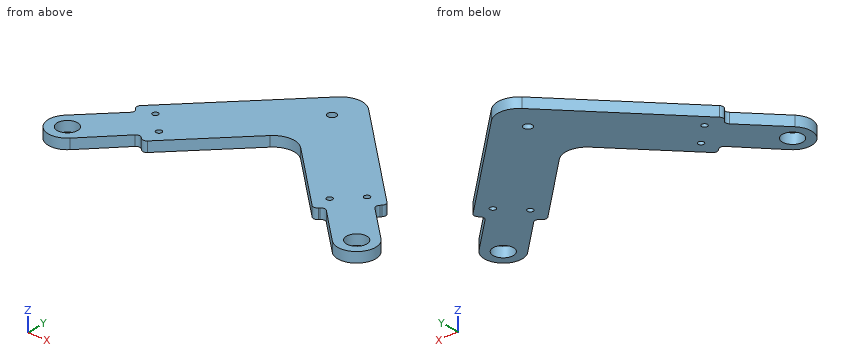
```python
from build123d import *

# Parameters (mm, degrees)
SKETCH7_R           = 3.5
SKETCH7_R_2         = 1
SKETCH7_R_3         = 1.5
BOSS_EXTRUDE1_DEPTH = 3.5
FILLET1_R           = 7.5
FILLET2_R           = 7.5
FILLET3_R           = 1.5
FILLET4_R           = 1.5
FILLET5_R           = 1.5


with BuildPart() as part:
    # Sketch7 → Boss-Extrude1 (new body)
    with BuildSketch(Plane.XY):
        with BuildLine():
            Line((-91.161165235, 18.03122292), (-104.596194078, 4.596194078))
            ThreePointArc((-104.596194078, 4.596194078), (-104.565177968, -4.627002282), (-95.342398812, -4.533955357))
            Line((-95.342398812, -4.533955357), (-82.149090724, 9.019148409))
            Line((-82.149090724, 9.019148409), (-79.493903346, 6.363961031))
            Line((-79.493903346, 6.363961031), (-50, 35.857864376))
            Line((-50, 35.857864376), (-20.445483687, 6.303348063))
            Line((-20.445483687, 6.303348063), (-17.970609953, 8.778221797))
            Line((-17.970609953, 8.778221797), (-4.596194078, -4.596194078))
            ThreePointArc((-4.596194078, -4.596194078), (4.596194078, -4.596194078), (4.596194078, 4.596194078))
            Line((4.596194078, 4.596194078), (-8.778221797, 17.970609953))
            Line((-8.778221797, 17.970609953), (-6.303348063, 20.445483687))
            Line((-6.303348063, 20.445483687), (-50, 64.142135624))
            Line((-50, 64.142135624), (-93.636038969, 20.506096654))
            Line((-93.636038969, 20.506096654), (-91.161165235, 18.03122292))
        make_face()
        Circle(SKETCH7_R, mode=Mode.SUBTRACT)
        with Locations((-100, 0)):
            Circle(SKETCH7_R, mode=Mode.SUBTRACT)
        with Locations((-86.564971157, 20.506096654)):
            Circle(SKETCH7_R_2, mode=Mode.SUBTRACT)
        with Locations((-50, 50)):
            Circle(SKETCH7_R_3, mode=Mode.SUBTRACT)
        with Locations((-13.374415875, 20.445483687)):
            Circle(SKETCH7_R_2, mode=Mode.SUBTRACT)
        with Locations((-20.445483687, 13.374415875)):
            Circle(SKETCH7_R_2, mode=Mode.SUBTRACT)
        with Locations((-79.493903346, 13.435028843)):
            Circle(SKETCH7_R_2, mode=Mode.SUBTRACT)
    extrude(amount=BOSS_EXTRUDE1_DEPTH)

    # Fillet1
    fillet1_edges = [part.edges().sort_by_distance(p)[0] for p in [
        (-50, 64.142135624, 1.75),
    ]]
    fillet(fillet1_edges, radius=FILLET1_R)

    # Fillet2
    fillet2_edges = [part.edges().sort_by_distance(p)[0] for p in [
        (-50, 35.857864376, 1.75),
    ]]
    fillet(fillet2_edges, radius=FILLET2_R)

    # Fillet3
    fillet3_edges = [part.edges().sort_by_distance(p)[0] for p in [
        (-82.149090724, 9.019148409, 1.75),
        (-93.636038969, 20.506096654, 1.75),
        (-17.970609953, 8.778221797, 1.75),
        (-20.445483687, 6.303348063, 1.75),
        (-79.493903346, 6.363961031, 1.75),
    ]]
    fillet(fillet3_edges, radius=FILLET3_R)

    # Fillet4
    fillet4_edges = [part.edges().sort_by_distance(p)[0] for p in [
        (-6.303348063, 20.445483687, 1.75),
        (-8.778221797, 17.970609953, 1.75),
    ]]
    fillet(fillet4_edges, radius=FILLET4_R)

    # Fillet5
    fillet5_edges = [part.edges().sort_by_distance(p)[0] for p in [
        (-91.161165235, 18.03122292, 1.75),
    ]]
    fillet(fillet5_edges, radius=FILLET5_R)


solid = part.part
```
Part model, mm, in its own coordinate system. Round coordinates to 2 decimals unless told otherwise and drop trailing zeros. Loops run counter-clockwise (first coordinate to the right, second up) from the corner with the lowest first, then second, coordinate; pieces in that order, holes last.
Item 1: Cut at D-D, the plane y = 37. Give the cut face in (x, z).
Item 2: Cut at C-C, the plane y = 50. Give the cut face in (x, z), then the cut area to 3 significant figures.
Item 3: Cut at B-B, the plane z = 1.9. State how many separate pieces and enclosed holes the cut face has, then the cut area to 3 significant figures.
Item 4: Drill centre lines: line 1 (X direction, y = 0.5, z = 1.45); line 2 (Y direction, x = -50, z = 1.9); line 3 (X direction, y = -2.5, z = 0.6). Where is each one in solid material? Low to high.
Item 5: Drop flat-ended pins along their axis: P1, Ø2, axis at x = -37, z = 0.5, coming from the +Y side; P2, Ø2, axis at y = 33.5, z = 3, coming from the +X side; P3, Ø2, axis at x = -86, z = 2, coming from the -Y side. Give the stop position or say it passes through.
Item 6: Cut at A-A, the plane x = -50. Give the cut face in (y, z), then the cut area to 3 significant figures.
A:
1. outline: (-77.14, 0) - (-22.86, 0) - (-22.86, 3.5) - (-77.14, 3.5) - close
2. outline: (-64.14, 0) - (-51.5, 0) - (-51.5, 3.5) - (-64.14, 3.5) - close; (-48.5, 0) - (-35.86, 0) - (-35.86, 3.5) - (-48.5, 3.5) - close
2. area: 88.5 mm2
3. separate pieces: 1
3. enclosed holes: 7
3. area: 2,600 mm2
4. line 1: x = -106.48 to -103.46, -96.54 to -90.44, -9.69 to -3.46, 3.46 to 6.48
4. line 2: y = 32.75 to 48.5, 51.5 to 61.04
4. line 3: x = -106 to -102.45, -97.55 to -93.36, -6.69 to -2.45, 2.45 to 6
5. P1: stops at y = 52.14
5. P2: stops at x = -18.36
5. P3: stops at y = 4.04
6. outline: (32.75, 0) - (48.5, 0) - (48.5, 3.5) - (32.75, 3.5) - close; (51.5, 0) - (61.04, 0) - (61.04, 3.5) - (51.5, 3.5) - close
6. area: 88.5 mm2
